Study the drawing (mm; zero at the part's minimum x, y, z) and answer. A direction names the side the tool comes from. Coordinates: 2 decimals unless noted, no trailing zeros. Order: outer loops, then holes, each group sorted by start corner. A loop starts at its lowest first (then second) coordinate and runs counter-clockwise, first axis right, second up.
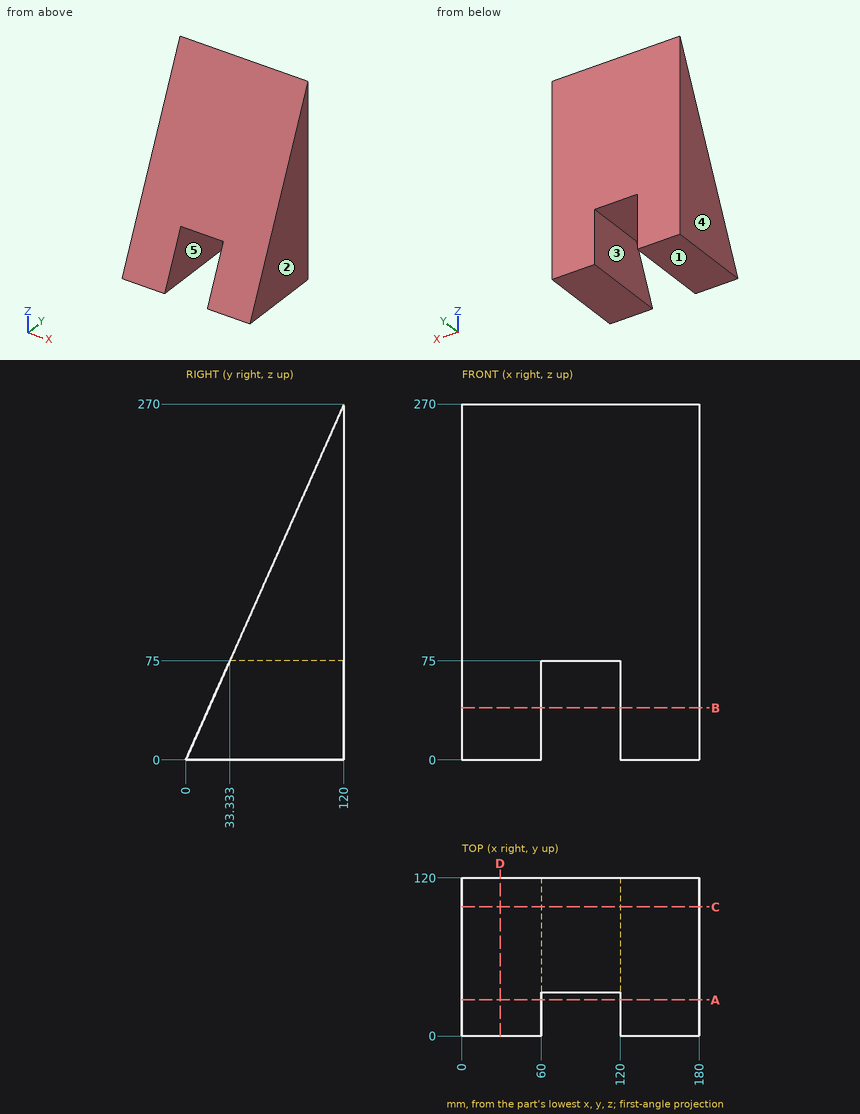
(1) Consider line 1 (X direction, y = 36, z = 18.5); line 2 (Z direction, x = 49.5, y = 103); line 3 (Y direction, x = 149, z = 222). Determine where each line is inside the solid, lowest interval first.
(2) For the marked faces 4 and 5, determine the directions among +Z, -Z, +X, -X, +Y, -Y from which every point of the face is accessible in a straight line to the end or side of a thin tool.
(3) Find section D-D (x = 29). Write down the section's boundary in (y, z), and give its area (3 significant figures).
(4) The mould has two halves that part along X. Classify the marked faces 1, 2 and 3: released by +X, released by -X, zero draft, split by the parting line, or undercut.
(5) Find section B-B (z = 39.5). Write down the section's boundary in (x, y) (1 decimal).
(6) Find section C-C (y = 98). Write down the section's boundary in (x, z).
(7) Find section A-A (y = 27.5). Write down the section's boundary in (x, z) (1 decimal), and give its area (4 significant figures).
(8) Each of these flat-tipped pins is pushed along its axis until it touches: pin 1 Ø6 at (x, z) = (99.5, 187.5) entering from -Y; pin 2 Ø6 at (x, y) = (29, 41) entering from +Z; pin 3 Ø1.5 at (x, z) = (97.5, 159) entering from -Y. Where does it stop, or does it pass through?
Findings below:
1. line 1: x = 0 to 60, 120 to 180
1. line 2: z = 0 to 231.75
1. line 3: y = 98.67 to 120
2. face 4: +Z, -Z, -X, +Y, -Y
2. face 5: -Z, +Y, -Y
3. outline: (0, 0) - (120, 0) - (120, 270) - close
3. area: 16,200 mm2
4. face 1: zero draft
4. face 2: released by +X
4. face 3: undercut
5. outline: (0, 17.6) - (60, 17.6) - (60, 120) - (0, 120) - close; (120, 17.6) - (180, 17.6) - (180, 120) - (120, 120) - close
6. outline: (0, 0) - (60, 0) - (60, 75) - (120, 75) - (120, 0) - (180, 0) - (180, 220.5) - (0, 220.5) - close
7. outline: (0, 0) - (60, 0) - (60, 61.9) - (0, 61.9) - close; (120, 0) - (180, 0) - (180, 61.9) - (120, 61.9) - close
7. area: 7,425 mm2
8. pin 1: stops at y = 82
8. pin 2: stops at z = 99
8. pin 3: stops at y = 70.33
